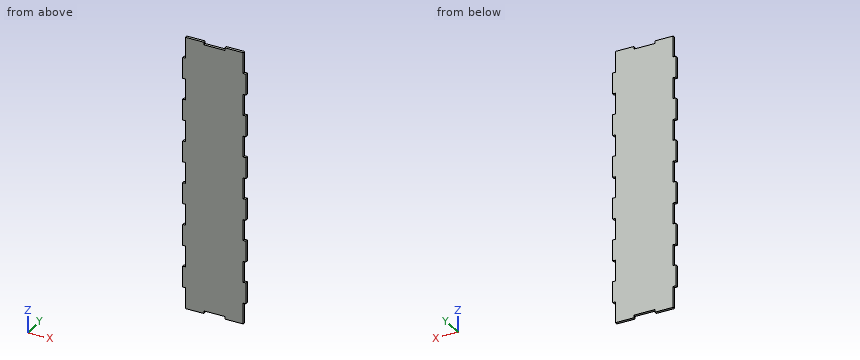
from build123d import *

# Parameters (mm, degrees)
BOSS_EXTRUDE1_DEPTH = 3.175
MIRROR1_START       = -161.925
MIRROR1_OUTLINE_W   = 69.85
MIRROR1_OUTLINE_H   = 3.175
MIRROR1_DEPTH       = 323.85
MIRROR1_START_2     = -165.1
MIRROR1_2_OUTLINE_W = 22.225
MIRROR1_2_OUTLINE_H = 3.175
MIRROR1_2_DEPTH     = 330.2
MIRROR1_START_3     = 12.7
MIRROR1_3_OUTLINE_W = 3.175
MIRROR1_3_OUTLINE_H = 3.175
MIRROR1_3_DEPTH     = 25.4
MIRROR1_START_4     = 63.5
MIRROR1_4_OUTLINE_W = 3.175
MIRROR1_4_OUTLINE_H = 3.175
MIRROR1_4_DEPTH     = 25.4
MIRROR1_START_5     = 114.3
MIRROR1_5_OUTLINE_W = 3.175
MIRROR1_5_OUTLINE_H = 3.175
MIRROR1_5_DEPTH     = 25.4
MIRROR1_START_6     = -139.7
MIRROR1_6_OUTLINE_W = 3.175
MIRROR1_6_OUTLINE_H = 3.175
MIRROR1_6_DEPTH     = 25.4
MIRROR1_START_7     = -88.9
MIRROR1_7_OUTLINE_W = 3.175
MIRROR1_7_OUTLINE_H = 3.175
MIRROR1_7_DEPTH     = 25.4
MIRROR1_START_8     = -38.1
MIRROR1_8_OUTLINE_W = 3.175
MIRROR1_8_OUTLINE_H = 3.175
MIRROR1_8_DEPTH     = 25.4


# Read off the part's stored shape, not the designer's step: Mirror1
with BuildPart() as part:
    # Sketch1 → Boss-Extrude1 (new body)
    with BuildSketch(Plane(origin=(0, 0, 0), x_dir=(1, 0, 0), z_dir=(0, 1, 0))):
        Polygon((0, 0), (0, 161.925), (-12.7, 161.925), (-12.7, 165.1), (-34.925, 165.1), (-34.925, 139.7), (-38.1, 139.7), (-38.1, 114.3), (-34.925, 114.3), (-34.925, 88.9), (-38.1, 88.9), (-38.1, 63.5), (-34.925, 63.5), (-34.925, 38.1), (-38.1, 38.1), (-38.1, 12.7), (-34.925, 12.7), (-34.925, 0), align=None)
    extrude(amount=BOSS_EXTRUDE1_DEPTH)

    # Mirror1 outline → Mirror1 (add)
    with BuildSketch(Plane.XY.offset(MIRROR1_START)):
        with Locations((0, 1.5875)):
            Rectangle(MIRROR1_OUTLINE_W, MIRROR1_OUTLINE_H)
    extrude(amount=MIRROR1_DEPTH)

    # Mirror1 2 outline → Mirror1 2 (add)
    with BuildSketch(Plane.XY.offset(MIRROR1_START_2)):
        with Locations((-23.8125, 1.5875)):
            Rectangle(MIRROR1_2_OUTLINE_W, MIRROR1_2_OUTLINE_H)
        with Locations((23.8125, 1.5875)):
            Rectangle(MIRROR1_2_OUTLINE_W, MIRROR1_2_OUTLINE_H)
    extrude(amount=MIRROR1_2_DEPTH)

    # Mirror1 3 outline → Mirror1 3 (add)
    with BuildSketch(Plane.XY.offset(MIRROR1_START_3)):
        with Locations((-36.5125, 1.5875)):
            Rectangle(MIRROR1_3_OUTLINE_W, MIRROR1_3_OUTLINE_H)
        with Locations((36.5125, 1.5875)):
            Rectangle(MIRROR1_3_OUTLINE_W, MIRROR1_3_OUTLINE_H)
    extrude(amount=MIRROR1_3_DEPTH)

    # Mirror1 4 outline → Mirror1 4 (add)
    with BuildSketch(Plane.XY.offset(MIRROR1_START_4)):
        with Locations((-36.5125, 1.5875)):
            Rectangle(MIRROR1_4_OUTLINE_W, MIRROR1_4_OUTLINE_H)
        with Locations((36.5125, 1.5875)):
            Rectangle(MIRROR1_4_OUTLINE_W, MIRROR1_4_OUTLINE_H)
    extrude(amount=MIRROR1_4_DEPTH)

    # Mirror1 5 outline → Mirror1 5 (add)
    with BuildSketch(Plane.XY.offset(MIRROR1_START_5)):
        with Locations((-36.5125, 1.5875)):
            Rectangle(MIRROR1_5_OUTLINE_W, MIRROR1_5_OUTLINE_H)
        with Locations((36.5125, 1.5875)):
            Rectangle(MIRROR1_5_OUTLINE_W, MIRROR1_5_OUTLINE_H)
    extrude(amount=MIRROR1_5_DEPTH)

    # Mirror1 6 outline → Mirror1 6 (add)
    with BuildSketch(Plane.XY.offset(MIRROR1_START_6)):
        with Locations((36.5125, 1.5875)):
            Rectangle(MIRROR1_6_OUTLINE_W, MIRROR1_6_OUTLINE_H)
    extrude(amount=MIRROR1_6_DEPTH)

    # Mirror1 7 outline → Mirror1 7 (add)
    with BuildSketch(Plane.XY.offset(MIRROR1_START_7)):
        with Locations((36.5125, 1.5875)):
            Rectangle(MIRROR1_7_OUTLINE_W, MIRROR1_7_OUTLINE_H)
    extrude(amount=MIRROR1_7_DEPTH)

    # Mirror1 8 outline → Mirror1 8 (add)
    with BuildSketch(Plane.XY.offset(MIRROR1_START_8)):
        with Locations((36.5125, 1.5875)):
            Rectangle(MIRROR1_8_OUTLINE_W, MIRROR1_8_OUTLINE_H)
    extrude(amount=MIRROR1_8_DEPTH)


solid = part.part
CAD build for the part. Positions are in the model's coordinates, mm. Give positions to 0.01 mm unless a question says otherwise; leave off trailing zeros. Loops run counter-clockwise (first coordinate to the right, second up) from the corner with the lowest first, then second, coordinate; pieces in that order, holes last. Notation, with made-up numbers: M 20,-36.5 L 40,-36.5 A20 ccw 40,1.5 Z; hole C 28.5,-40 d10. An arc over 180 degrees is marked long. Answer in a Markdown table with one row per item. Add a question column.
Item 1: Probe probe 1 along X at (y, z) = (0.75, -48) (3 decimals); probe 2 along Z at (x, y) = (-3.5, 2.85) (3 decimals). List the from-to ranges inside material, lowest first.
Item 2: Band-saw the part on B-B on x = -9. Give the cut face in (y, z) (3 decimals).
Item 3: Drop flat-ended pins along their axis: P1, Ø1, axis at x = -37, y = 1, coming from the +Z side; P2, Ø1, axis at y = 2, z = -163, coming from the -X side (3 decimals); P3, Ø12, axis at x = 1.5, z = -29.5, coming from the -Y side; P4, Ø1, axis at x = -36.5, y = 1.5, coming from the -Z side. Give the stop position or say it passes through.
Item 4: Band-saw the part on A-A on z = 45. Give the cut face in (x, y) (3 decimals), then the cut area to 3 significant figures.
Reply:
| question | item | result |
|---|---|---|
| 1 | probe 1 | x = -34.925 to 34.925 |
| 1 | probe 2 | z = -161.925 to 161.925 |
| 2 | outline | M 0,-161.925 L 3.175,-161.925 L 3.175,161.925 L 0,161.925 Z |
| 3 | P1 | stops at z = 139.7 |
| 3 | P2 | stops at x = -34.925 |
| 3 | P3 | stops at y = 0 |
| 3 | P4 | stops at z = -139.7 |
| 4 | outline | M -34.925,0 L 34.925,0 L 34.925,3.175 L -34.925,3.175 Z |
| 4 | area | 222 mm^2 |
